Can you work these out from the model? Positions are in its coordinate system, mm. Give positions to 0.01 mm unless a question says otherwise; leave off trailing zeros. Loops run counter-clockwise (first coordinate to the right, second up) from the corner with the lowest first, then second, coordinate; pieces in that order, holes last. Notation, with made-up numbers: (21, 60) - (69, 60) arc R23 ccw to (69, 88) - close; hole circle Ø9 at (72.25, -39.5). An arc over 180 degrees is marked (long way). Answer in a Markdown table with one row per item.
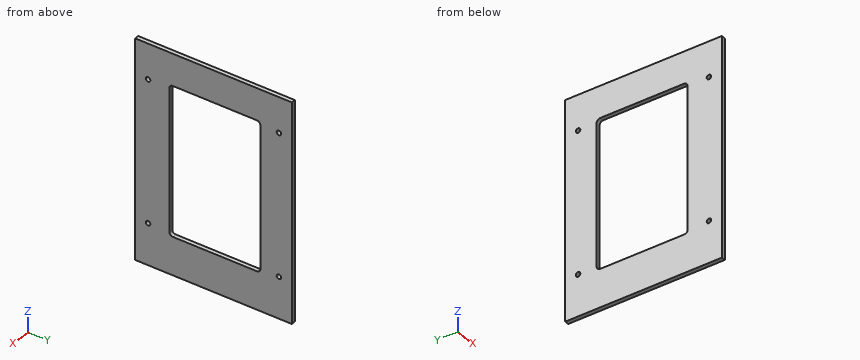
Autodesk Inventor part; units mm, degrees
ref_plane "YZ Plane" through (0, 0, 0) normal (1, 0, 0) x (0, 1, 0)
ref_plane "XZ Plane" through (0, 0, 0) normal (0, 1, 0) x (-1, 0, 0)
ref_plane "XY Plane" through (0, 0, 0) normal (0, 0, 1) x (1, 0, 0)
sketch "Face" plane through (0, 0, 0) normal (0, 0, 1) x (1, 0, 0)
  line L0 (38.5, 208.87) -> (135.1, 208.87)
  arc A0 (38.5, 208.87) -> (34.5, 204.87) centre (38.5, 204.87) ccw
  circle A1 centre (10, 204.87) radius 2.6
  line L1 (175.25, 245.25) -> (-4.75, 245.25)
  line L2 (139.1, 204.87) -> (139.1, 42.67)
  line L3 (34.5, 42.67) -> (34.5, 204.87)
  line L4 (175.25, -4.75) -> (175.25, 245.25)
  line L5 (-4.75, 245.25) -> (-4.75, -4.75)
  circle A2 centre (160.5, 42.67) radius 2.6
  arc A3 (135.1, 38.67) -> (139.1, 42.67) centre (135.1, 42.67) ccw
  arc A4 (34.5, 42.67) -> (38.5, 38.67) centre (38.5, 42.67) ccw
  circle A5 centre (10, 42.67) radius 2.6
  line L6 (-4.75, -4.75) -> (175.25, -4.75)
  line L7 (135.1, 38.67) -> (38.5, 38.67)
  arc A6 (139.1, 204.87) -> (135.1, 208.87) centre (135.1, 204.87) ccw
  circle A7 centre (160.5, 204.87) radius 2.6
  point P0 (84.3959, 120.382)
  point P1 (0, 0)
sketch "Sketch1" plane through (0, 0, 0) normal (1, 0, 0) x (0, 1, 0)
  line L0 (-46.75, 88.62) -> (49.85, 88.62)
  arc A0 (-46.75, 88.62) -> (-50.75, 84.62) centre (-46.75, 84.62) ccw
  circle A1 centre (-75.25, 84.62) radius 2.6
  line L1 (90, 125) -> (-90, 125)
  line L2 (53.85, 84.62) -> (53.85, -77.58)
  line L3 (-50.75, -77.58) -> (-50.75, 84.62)
  line L4 (90, -125) -> (90, 125)
  line L5 (-90, 125) -> (-90, -125)
  circle A2 centre (75.25, -77.58) radius 2.6
  arc A3 (49.85, -81.58) -> (53.85, -77.58) centre (49.85, -77.58) ccw
  arc A4 (-50.75, -77.58) -> (-46.75, -81.58) centre (-46.75, -77.58) ccw
  circle A5 centre (-75.25, -77.58) radius 2.6
  line L6 (-90, -125) -> (90, -125)
  line L7 (49.85, -81.58) -> (-46.75, -81.58)
  arc A6 (53.85, 84.62) -> (49.85, 88.62) centre (49.85, 84.62) ccw
  circle A7 centre (75.25, 84.62) radius 2.6
  point P0 (0, 0)
  point P1 (0, 125)
  point P2 (90, 0)
extrude "Extrusion1" add sketch "Sketch1" along normal mid plane 4.75
properties part number "BREEZE-M06"
Q1. For pin 1 (4.5 mm diameter, centred on y = -75.25, z = -77.58, fed in from +X), with a flat end and sliding along its axis, tell me the tip position at first contact or that it passes through.
Checked values:
| item | result |
|---|---|
| pin 1 | passes through |
Q2. Imagine slicing it at C-C, the plane x = -1.3. Write out the boundary of the cut face in (y, z), and give its area (3 significant figures).
Checked values:
| item | result |
|---|---|
| outline | (-90, -125) - (90, -125) - (90, 125) - (-90, 125) - close; hole circle Ø5.2 at (-75.25, -77.58); hole circle Ø5.2 at (-75.25, 84.62); hole (-50.75, -77.58) arc R4 ccw to (-46.75, -81.58) - (49.85, -81.58) arc R4 ccw to (53.85, -77.58) - (53.85, 84.62) arc R4 ccw to (49.85, 88.62) - (-46.75, 88.62) arc R4 ccw to (-50.75, 84.62) - close; hole circle Ø5.2 at (75.25, -77.58); hole circle Ø5.2 at (75.25, 84.62) |
| area | 27,100 mm² |
Q3. Imagine slicing it at A-A, the plane y = -75.25. Write out the boundary of the cut face in (x, z) (3 decimals).
Checked values:
| item | result |
|---|---|
| outline | (-2.375, -125) - (2.375, -125) - (2.375, -80.18) - (-2.375, -80.18) - close; (-2.375, -74.98) - (2.375, -74.98) - (2.375, 82.02) - (-2.375, 82.02) - close; (-2.375, 87.22) - (2.375, 87.22) - (2.375, 125) - (-2.375, 125) - close |
Q4. If I drill on line 1 (Z direction, x = -0.5, y = 75.25); line 2 (Z direction, x = 0.85, y = -11.5); line 3 (Y direction, x = -0.2, z = -10.5), over which ranges is the centre line in solid material (lowest first)? Write a range as [from, to].
Checked values:
| item | result |
|---|---|
| line 1 | z = [-125, -80.18], [-74.98, 82.02], [87.22, 125] |
| line 2 | z = [-125, -81.58], [88.62, 125] |
| line 3 | y = [-90, -50.75], [53.85, 90] |
Q5. Imagine slicing it at B-B, the plane z = -65. Write out the boundary of the cut face in (x, y) (3 decimals), and give its area (3 significant figures).
Checked values:
| item | result |
|---|---|
| outline | (-2.375, -90) - (2.375, -90) - (2.375, -50.75) - (-2.375, -50.75) - close; (-2.375, 53.85) - (2.375, 53.85) - (2.375, 90) - (-2.375, 90) - close |
| area | 358 mm² |
Q6. Imagine slicing it at D-D, the plane y = -0.5. Write out the boundary of the cut face in (x, z) (3 decimals).
Checked values:
| item | result |
|---|---|
| outline | (-2.375, -125) - (2.375, -125) - (2.375, -81.58) - (-2.375, -81.58) - close; (-2.375, 88.62) - (2.375, 88.62) - (2.375, 125) - (-2.375, 125) - close |
